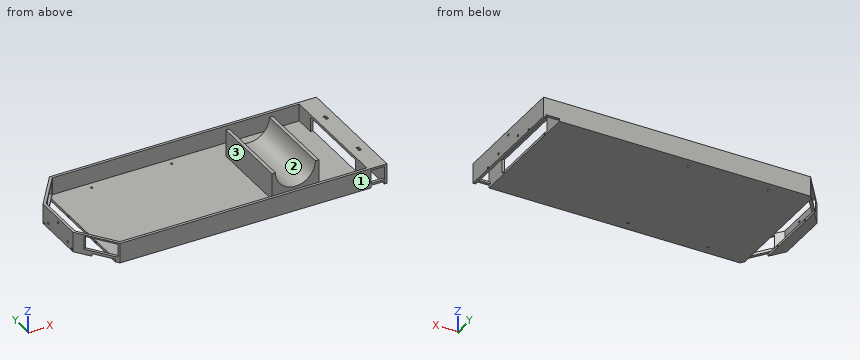
from build123d import *

# Parameters (mm, degrees)
F0_W      = 254
F0_H      = 119.38
F1_DEPTH  = 19.05
F2_T      = -2.54
F3_W      = 30.48
F3_H      = 12.7
F4_DEPTH  = 2.54
F5_W      = 12.7
F5_H      = 119.38
F6_DEPTH  = 2.54
F7_R      = 1.016
F8_DEPTH  = 25.4
F9_R      = 1.016
F10_DEPTH = 25.4
F11_W     = 30.48
F11_H     = 12.7
F12_DEPTH = 2.54
F13_W     = 12.7
F13_H     = 12.7
F14_DEPTH = 101.6
F15_R     = 1.1176
F16_DEPTH = 84.582
F17_R     = 1.1176
F18_DEPTH = 279.4
F20_DEPTH = 2.54
F21_W     = 44.45
F21_H     = 77.978
F22_DEPTH = 25.4
F23_R     = 19
F24_DEPTH = 77.978
F25_W     = 114.3
F25_H     = 1.905
F26_DEPTH = 12.7
F27_W     = 2.54
F27_H     = 114.3
F28_DEPTH = 16.51
F29_W     = 2.54
F29_H     = 5.08
F30_DEPTH = 25.4
F31_W     = 76.2
F31_H     = 13.97
F32_DEPTH = 5.08


with BuildPart() as f1:
    # F0 (on Top) → F1 (new body)
    with BuildSketch(Plane.XY):
        Rectangle(F0_W, F0_H)
        Polygon((-152.4, -25.4), (-127, -59.69), (-127, 59.69), (-152.4, 25.4), align=None)
    extrude(amount=F1_DEPTH)

    # F2
    f2_openings = [f1.faces().sort_by_distance(p)[0] for p in [
        (-9.181331, 0, 19.05),
    ]]
    offset(amount=F2_T, openings=f2_openings)

    # F3 (on face) → F4 (cut)
    with BuildSketch(Plane(origin=(-110.5541186891, -81.8919397697, 0), x_dir=(0.5952275506, -0.8035571933, 0), z_dir=(-0.8035571933, -0.5952275506, 0))):
        with Locations((-44.9023260044, 11.43)):
            Rectangle(F3_W, F3_H)
    extrude(amount=-F4_DEPTH, mode=Mode.SUBTRACT)

    # F5 (on face) → F6 (cut)
    with BuildSketch(Plane(origin=(0, 0, 0), x_dir=(1, 0, 0), z_dir=(0, 0, -1))):
        Polygon((-129.54, -56.261), (-129.54, 56.261), (-142.24, 39.116), (-142.24, -39.116), align=None)
        with Locations((118.11, 0)):
            Rectangle(F5_W, F5_H)
    extrude(amount=-F6_DEPTH, mode=Mode.SUBTRACT)

    # F7 (on face) → F8 (cut)
    with BuildSketch(Plane(origin=(-152.4, 0, 0), x_dir=(0, -1, 0), z_dir=(-1, 0, 0))):
        with Locations((-23.114, 1.27)):
            Circle(F7_R)
        with Locations((23.114, 1.27)):
            Circle(F7_R)
    extrude(amount=-F8_DEPTH, mode=Mode.SUBTRACT)

    # F9 (on face) → F10 (cut)
    with BuildSketch(Plane.YZ.offset(127)):
        with Locations((-34.29, 1.27)):
            Circle(F9_R)
        with Locations((34.29, 1.27)):
            Circle(F9_R)
    extrude(amount=-F10_DEPTH, mode=Mode.SUBTRACT)

    # F11 (on face) → F12 (cut)
    with BuildSketch(Plane(origin=(-110.5541186891, 81.8919397697, 0), x_dir=(-0.5952275506, -0.8035571933, 0), z_dir=(-0.8035571933, 0.5952275506, 0))):
        with Locations((44.9023260044, 10.16)):
            Rectangle(F11_W, F11_H)
    extrude(amount=-F12_DEPTH, mode=Mode.SUBTRACT)

    # F13 (on face) → F14 (cut)
    with BuildSketch(Plane.XZ.offset(59.69)):
        with Locations((118.11, 10.795)):
            Rectangle(F13_W, F13_H)
    extrude(amount=-F14_DEPTH, mode=Mode.SUBTRACT)

    # F15 (on Right) → F16 (cut, symmetric)
    with BuildSketch(Plane.YZ):
        with Locations((0, 11.811)):
            Circle(F15_R)
        with Locations((-17.78, 5.08)):
            Circle(F15_R)
        with Locations((17.78, 5.08)):
            Circle(F15_R)
    extrude(amount=F16_DEPTH, both=True, mode=Mode.SUBTRACT)

    # F17 (on face) → F18 (cut)
    with BuildSketch(Plane(origin=(-152.4, 0, 0), x_dir=(0, -1, 0), z_dir=(-1, 0, 0))):
        with Locations((-16.4471499023, 5.0268133191)):
            Circle(F17_R)
        with Locations((16.4471499023, 5.0268133191)):
            Circle(F17_R)
        with Locations((0, 14.5379047776)):
            Circle(F17_R)
    extrude(amount=-F18_DEPTH, mode=Mode.SUBTRACT)

    # F19 (on face) → F20 (cut)
    with BuildSketch(Plane.XY.offset(2.54)):
        with BuildLine():
            Line((-91.8904091179, -50.8), (-90.7728091179, -50.8))
            ThreePointArc((-90.7728091179, -50.8), (-91.1001465793, -50.0097374613), (-91.8904091179, -49.6824))
            Line((-91.8904091179, -49.6824), (-91.8904091179, -50.8))
        make_face()
        with BuildLine():
            ThreePointArc((-91.8904091179, -49.6824), (-92.6806716566, -51.5902625387), (-90.7728091179, -50.8))
            Line((-90.7728091179, -50.8), (-91.8904091179, -50.8))
            Line((-91.8904091179, -50.8), (-91.8904091179, -49.6824))
        make_face()
        with BuildLine():
            Line((-15.6904091179, -50.8), (-16.8080091179, -50.8))
            ThreePointArc((-16.8080091179, -50.8), (-15.6904091179, -51.9176), (-14.5728091179, -50.8))
            ThreePointArc((-14.5728091179, -50.8), (-14.9001465793, -50.0097374613), (-15.6904091179, -49.6824))
            Line((-15.6904091179, -49.6824), (-15.6904091179, -50.8))
        make_face()
        with BuildLine():
            ThreePointArc((-15.6904091179, -49.6824), (-16.4806716566, -50.0097374613), (-16.8080091179, -50.8))
            Line((-16.8080091179, -50.8), (-15.6904091179, -50.8))
            Line((-15.6904091179, -50.8), (-15.6904091179, -49.6824))
        make_face()
        with BuildLine():
            Line((-15.6904091179, 50.8), (-15.6904091179, 49.6824))
            ThreePointArc((-15.6904091179, 49.6824), (-14.9001465793, 50.0097374613), (-14.5728091179, 50.8))
            ThreePointArc((-14.5728091179, 50.8), (-15.6904091179, 51.9176), (-16.8080091179, 50.8))
            Line((-16.8080091179, 50.8), (-15.6904091179, 50.8))
        make_face()
        with BuildLine():
            ThreePointArc((-16.8080091179, 50.8), (-16.4806716566, 50.0097374613), (-15.6904091179, 49.6824))
            Line((-15.6904091179, 49.6824), (-15.6904091179, 50.8))
            Line((-15.6904091179, 50.8), (-16.8080091179, 50.8))
        make_face()
        with BuildLine():
            ThreePointArc((-90.7728091179, 50.8), (-92.6806716566, 51.5902625387), (-91.8904091179, 49.6824))
            Line((-91.8904091179, 49.6824), (-91.8904091179, 50.8))
            Line((-91.8904091179, 50.8), (-90.7728091179, 50.8))
        make_face()
        with BuildLine():
            Line((-91.8904091179, 50.8), (-91.8904091179, 49.6824))
            ThreePointArc((-91.8904091179, 49.6824), (-91.1001465793, 50.0097374613), (-90.7728091179, 50.8))
            Line((-90.7728091179, 50.8), (-91.8904091179, 50.8))
        make_face()
    extrude(amount=-F20_DEPTH, mode=Mode.SUBTRACT)

    # F21 (on face) → F22 (join)
    with BuildSketch(Plane.XY.offset(2.54)):
        with Locations((51.5379719436, 0)):
            Rectangle(F21_W, F21_H)
    extrude(amount=F22_DEPTH)

    # F23 (on face) → F24 (cut)
    with BuildSketch(Plane.XZ.offset(38.989)):
        with Locations((51.5379719436, 27.94)):
            Circle(F23_R)
    extrude(amount=-F24_DEPTH, mode=Mode.SUBTRACT)

    # F25 (on face) → F26 (join)
    with BuildSketch(Plane(origin=(124.46, 0, 0), x_dir=(0, -1, 0), z_dir=(-1, 0, 0))):
        with Locations((0, 18.0975)):
            Rectangle(F25_W, F25_H)
    extrude(amount=F26_DEPTH)

    # F27 (on face) → F28 (join)
    with BuildSketch(Plane.XY.offset(2.54)):
        with Locations((110.49, 0)):
            Rectangle(F27_W, F27_H)
    extrude(amount=F28_DEPTH)

    # F29 (on face) → F30 (cut)
    with BuildSketch(Plane.XY.offset(19.05)):
        with Locations((118.11, 27.94)):
            Rectangle(F29_W, F29_H)
        with Locations((118.11, -27.94)):
            Rectangle(F29_W, F29_H)
    extrude(amount=-F30_DEPTH, mode=Mode.SUBTRACT)

    # F31 (on face) → F32 (cut)
    with BuildSketch(Plane(origin=(109.22, 0, 0), x_dir=(0, -1, 0), z_dir=(-1, 0, 0))):
        with Locations((0, 9.525)):
            Rectangle(F31_W, F31_H)
    extrude(amount=-F32_DEPTH, mode=Mode.SUBTRACT)


solid = f1.part
For this review, take the finished solid that the model builds, in its own axes (mm). Face numbers are marked on the shaded views. Give positions to 0.01 mm unless a question says otherwise; leave off trailing zeros. Loops run counter-clockwise (first coordinate to the right, second up) from the corner with the lowest first, then second, coordinate; pieces in that order, holes last.
Item 1: Draft analysis for pull direction X (two halves, no side actions). For the marked faces 1, 2 and 3, state which applies: +X half, -X half, draft (parallel to the pull), parting line (faces both ways), or undercut.
Item 2: For line 1 along Y through (x, z) = (61.5, 10); line 2 along X through (y, z) = (50.8, 0.5); line 3 along X through (y, z) = (-14.5, 8.25), list the stretches that pass through material, from the lowest coordinate up.
Item 3: Take a section at C-C, the plane z = 22.25. State the section outline as (x, y) points, and give its area (3 significant figures).
Item 4: Insertion check: pin 1 (2 mm diameter, centred on x = 76.5, y = -20.5, fed in from +Z); pin 2 (6 mm diameter, centred on x = -139.5, y = 51, fed in from +Z); pin 3 (6 mm diameter, centred on x = -147, y = 14.5, fed in from +Z); pin 4 (5 mm diameter, centred on y = 28.5, z = 12, fed in from -X). Each pin has a flat end and moves straight along its axis. Give the tip position at first contact, or say it passes through.
Item 5: Take a section at D-D, the plane x = -134.5. State the section outline as (y, z) points (3 decimals), and give its area (3 significant figures).
Item 6: Take a section at A-A, the plane y = -5.5. State the section outline as (x, z) points (3 decimals), and give its area (3 significant figures).
Item 7: Take a section at B-B, the plane x = 86. State the section outline as (y, z) points, and give its area (3 significant figures).
Calculated:
1. face 1: draft
1. face 2: undercut
1. face 3: undercut
2. line 1: y = -59.69 to -57.15, -38.99 to 38.99, 57.15 to 59.69
2. line 2: x = -129.54 to -93.01, -90.77 to -16.81, -14.57 to 111.76, 124.46 to 127
2. line 3: x = -152.4 to -149.86, 29.31 to 73.76, 124.46 to 127
3. outline: (29.31, -38.99) - (33.41, -38.99) - (33.41, 38.99) - (29.31, 38.99) - close; (69.67, -38.99) - (73.76, -38.99) - (73.76, 38.99) - (69.67, 38.99) - close
3. area: 639 mm2
4. pin 1: stops at z = 2.54
4. pin 2: passes through
4. pin 3: stops at z = 19.05
4. pin 4: stops at x = -151.96
5. outline: (-49.565, 2.54) - (-45.298, 2.54) - (-45.298, 5.08) - (-49.565, 5.08) - close; (-49.565, 17.78) - (-45.298, 17.78) - (-45.298, 19.05) - (-49.565, 19.05) - close; (45.298, 2.54) - (49.565, 2.54) - (49.565, 3.81) - (45.298, 3.81) - close; (45.298, 16.51) - (49.565, 16.51) - (49.565, 19.05) - (45.298, 19.05) - close
5. area: 32.5 mm2
6. outline: (-152.4, 0) - (-142.24, 0) - (-142.24, 2.54) - (-149.86, 2.54) - (-149.86, 19.05) - (-152.4, 19.05) - close; (-129.54, 0) - (111.76, 0) - (111.76, 2.54) - (73.763, 2.54) - (73.763, 27.94) - (70.538, 27.94) arc R19 cw to (32.538, 27.94) - (29.313, 27.94) - (29.313, 2.54) - (-129.54, 2.54) - close; (109.22, 16.51) - (111.76, 16.51) - (111.76, 17.145) - (124.46, 17.145) - (124.46, 0) - (127, 0) - (127, 19.05) - (109.22, 19.05) - close
6. area: 1,320 mm2
7. outline: (-59.69, 0) - (59.69, 0) - (59.69, 19.05) - (57.15, 19.05) - (57.15, 2.54) - (-57.15, 2.54) - (-57.15, 19.05) - (-59.69, 19.05) - close
7. area: 387 mm2
